Read the model definition and answer for the solid it produces. Units are mm, in the model's axes. Face numbers are marked on the shaded views. A direction names the side the tool comes from. Coordinates: 2 decimals unless noted, no trailing zeros. Write each loop counter-clockwise with the first axis right and the second up, starting at its lowest first coordinate (ties: lowest second). Pieces come first, ordered by that corner, then holes. Notation, with made-up numbers: M 17.5,-12.5 L 61.5,-12.5 A8 cw 61.5,-2.5 Z; hole C 82.5,-19.5 d2. An arc over 180 degrees is marked long. Use a Markdown table: item, result. Add a question column.
from build123d import *

# Parameters (mm, degrees)
SKETCH1_W           = 24.634
SKETCH1_H           = 13
BOSS_EXTRUDE1_DEPTH = 10
SKETCH4_W           = 82.5
SKETCH4_H           = 13
BOSS_EXTRUDE4_DEPTH = 15
SKETCH5_W           = 28
SKETCH5_H           = 3.5
BOSS_EXTRUDE5_DEPTH = 15
CUT_EXTRUDE1_DEPTH  = 88.769584709
SKETCH7_W           = 28
SKETCH7_H           = 5
CUT_EXTRUDE2_DEPTH  = 2
SKETCH11_R          = 2.68
CUT_EXTRUDE3_DEPTH  = 88.769584709
FILLET1_R           = 10
FILLET2_R           = 5


with BuildPart() as part:
    # Sketch1 → Boss-Extrude1 (new body)
    with BuildSketch(Plane.XY):
        with Locations((12.317, 6.5)):
            Rectangle(SKETCH1_W, SKETCH1_H)
    extrude(amount=BOSS_EXTRUDE1_DEPTH)

    # Sketch4 → Boss-Extrude4 (add)
    with BuildSketch(Plane.XY.offset(10)):
        with Locations((41.25, 6.5)):
            Rectangle(SKETCH4_W, SKETCH4_H)
    extrude(amount=BOSS_EXTRUDE4_DEPTH)

    # Sketch5 → Boss-Extrude5 (add)
    with BuildSketch(Plane.XY.offset(25)):
        with Locations((68.5, -1.75)):
            Rectangle(SKETCH5_W, SKETCH5_H)
        with Locations((68.5, 14.75)):
            Rectangle(SKETCH5_W, SKETCH5_H)
    extrude(amount=-BOSS_EXTRUDE5_DEPTH)

    # Sketch6 → Cut-Extrude1 (cut, through all)
    with BuildSketch(Plane.XY.offset(25)):
        with BuildLine():
            Line((63.16, 9.16), (69.84, 9.16))
            ThreePointArc((69.84, 9.16), (72.5, 6.5), (69.84, 3.84))
            Line((69.84, 3.84), (63.16, 3.84))
            ThreePointArc((63.16, 3.84), (60.5, 6.5), (63.16, 9.16))
        make_face()
    extrude(amount=-CUT_EXTRUDE1_DEPTH, mode=Mode.SUBTRACT)

    # Sketch7 → Cut-Extrude2 (cut)
    with BuildSketch(Plane.XY.offset(25)):
        with Locations((68.5, 6.5)):
            Rectangle(SKETCH7_W, SKETCH7_H)
    extrude(amount=-CUT_EXTRUDE2_DEPTH, mode=Mode.SUBTRACT)

    # Sketch11 → Cut-Extrude3 (cut, through all)
    with BuildSketch(Plane(origin=(0, 0, 0), x_dir=(-1, 0, 0), z_dir=(0, 0, -1))):
        with Locations((-5.067, 6.5)):
            Circle(SKETCH11_R)
        with Locations((-19.567, 6.5)):
            Circle(SKETCH11_R)
    extrude(amount=-CUT_EXTRUDE3_DEPTH, mode=Mode.SUBTRACT)

    # Fillet1
    # the kernel refuses this fillet: 10 mm, written as the material it adds along each edge
    with BuildSketch(Plane(origin=(54.5, 13, 25), x_dir=(-1, 0, 0), z_dir=(0, 0, -1))) as fillet1_piece_1:
        with BuildLine():
            CenterArc((7.599342077, 10), FILLET1_R, 220.541601874, 49.458398126)
            Line((0, 3.5), (-0.151986842, 3.37))
            ThreePointArc((-0.151986842, 3.37), (-0.2, 1.75), (-0.2, 0))
            Line((-0.2, 0), (0, -0.2))
            Line((0, -0.2), (7.599342077, -0.2))
            Line((7.599342077, -0.2), (7.599342077, 0))
        make_face()
    extrude(amount=15)
    with BuildSketch(Plane(origin=(54.5, 0, 25), x_dir=(-1, 0, 0), z_dir=(0, 0, -1))) as fillet1_piece_2:
        with BuildLine():
            CenterArc((7.599342077, -10), FILLET1_R, 90, 49.458398126)
            Line((0, -3.5), (-0.151986842, -3.37))
            ThreePointArc((-0.151986842, -3.37), (-0.2, -1.75), (-0.2, 0))
            Line((-0.2, 0), (0, 0.2))
            Line((0, 0.2), (7.599342077, 0.2))
            Line((7.599342077, 0.2), (7.599342077, 0))
        make_face()
    extrude(amount=15)

    # Fillet2
    fillet2_edges = [part.edges().sort_by_distance(p)[0] for p in [
        (24.634, 6.5, 10),
    ]]
    fillet(fillet2_edges, radius=FILLET2_R)


solid = part.part
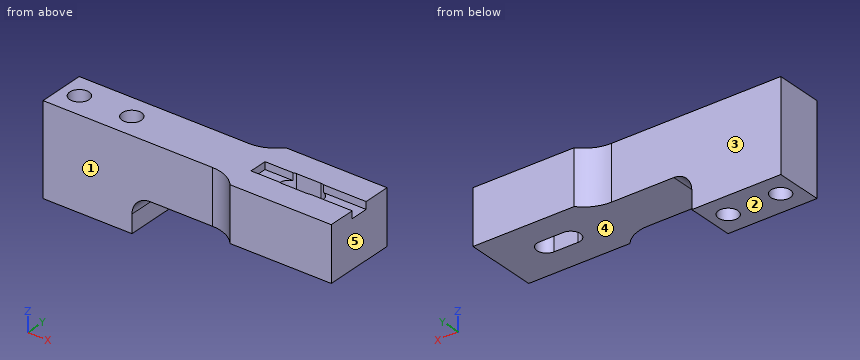
Item 1: For the marked faces 1, 2, 3, 4 and 5, determine the directions among +Z, -Z, +X, -X, +Y, -Y from which every point of the face is accessible in a straight line to the end or side of a thin tool.
Item 2: Consider probe 1 along Y at (x, z) = (69.5, 18.5); probe 2 along Z at (x, y) = (46, 12.75); probe 3 along X at (y, z) = (7, 8.25). Determine where each line is inside the solid, lowest interval first.
Item 3: Find section C-C on z = 13.25. Give the vertices of the cut face in (x, y), then the cut area to 3 significant figures.
Item 4: Find section D-D on y = 1.75. Give the vertices of the cut face in (x, z).
Item 5: Each of these flat-tipped pins is pushed along its axis until it touches: pin 1 (7.5 mm diameter, centred on x = 29, z = 16, fed in from +Y); pin 2 (2 mm diameter, centred on x = 41, y = 0.5, fed in from -Z); pin 3 (5 mm diameter, centred on x = 19.567, y = 6.5, fed in from +Z); pin 4 (6 mm diameter, centred on x = 5.067, y = 6.5, fed in from -Z). Where does it stop, or does it pass through?
Item 6: Find section B-B on x = 19. Give the vertices of the cut face in (y, z), then the cut area to 3 significant figures.
Item 7: Find section A-A on y = 6.5. Give the vertices of the cut face in (x, z), then the cut area to 3 significant figures.
Geometry says:
| question | item | result |
|---|---|---|
| 1 | face 1 | +Z, -Z, -X, -Y |
| 1 | face 2 | -Z, +X, -X, +Y, -Y |
| 1 | face 3 | +Z, -Z, -X, +Y |
| 1 | face 4 | -Z, +X, +Y, -Y |
| 1 | face 5 | +Z, -Z, +X, +Y, -Y |
| 2 | probe 1 | y = -3.5 to 3.84, 9.16 to 16.5 |
| 2 | probe 2 | z = 10 to 25 |
| 2 | probe 3 | x = 0 to 2.43, 7.7 to 16.93, 22.2 to 25.83 |
| 3 | outline | M 0,0 L 46.9,0 A10 cw 54.5,-3.5 L 82.5,-3.5 L 82.5,16.5 L 54.5,16.5 A10 cw 46.9,13 L 0,13 Z; hole C 5.07,6.5 d5.36; hole C 19.57,6.5 d5.36; hole M 63.16,3.84 L 69.84,3.84 A2.66 ccw 69.84,9.16 L 63.16,9.16 A2.66 ccw Z |
| 3 | area | 1,180 mm2 |
| 4 | outline | M 0,0 L 24.63,0 L 24.63,5 A5 cw 29.63,10 L 82.5,10 L 82.5,25 L 0,25 Z |
| 5 | pin 1 | stops at y = 13 |
| 5 | pin 2 | stops at z = 10 |
| 5 | pin 3 | passes through |
| 5 | pin 4 | stops at z = 0 |
| 6 | outline | M 0,0 L 3.88,0 L 3.88,25 L 0,25 Z; M 9.12,0 L 13,0 L 13,25 L 9.12,25 Z |
| 6 | area | 194 mm2 |
| 7 | outline | M 0,0 L 2.39,0 L 2.39,25 L 0,25 Z; M 7.75,0 L 16.89,0 L 16.89,25 L 7.75,25 Z; M 22.25,0 L 24.63,0 L 24.63,5 A5 cw 29.63,10 L 60.5,10 L 60.5,23 L 54.5,23 L 54.5,25 L 22.25,25 Z; M 72.5,10 L 82.5,10 L 82.5,23 L 72.5,23 Z |
| 7 | area | 1,010 mm2 |
